Autodesk Inventor part; units mm, degrees
ref_plane "YZ Plane" through (0, 0, 0) normal (1, 0, 0) x (0, 1, 0)
ref_plane "XZ Plane" through (0, 0, 0) normal (0, 1, 0) x (-1, 0, 0)
ref_plane "XY Plane" through (0, 0, 0) normal (0, 0, 1) x (1, 0, 0)
sketch "Sketch1" plane through (0, 0, 0) normal (0, 0, 1) x (1, 0, 0)
  arc A0 (-3.1, 0) -> (3.1, 0) centre (0, 0) ccw
  arc A1 (-5.5, 0) -> (5.5, 0) centre (0, 0) ccw
  line L0 (-3.1, 0) -> (-5.5, 0)
  line L1 (-5.5, 0) -> (-5.5, 5.5)
  line L2 (-5.5, 5.5) -> (-3.1, 5.5)
  line L3 (-3.1, 5.5) -> (-3.1, 0)
  line L4 (3.1, 0) -> (5.5, 0)
  line L5 (5.5, 0) -> (5.5, 5.5)
  line L6 (5.5, 5.5) -> (3.1, 5.5)
  line L7 (3.1, 5.5) -> (3.1, 0)
  line L8 (-5.5, 0) -> (-5.5, 5.5)
  line L9 (-5.5, 5.5) -> (-17.5, 5.5)
  line L10 (-17.5, 5.5) -> (-17.5, 0)
  line L11 (-17.5, 0) -> (-5.5, 0)
  line L12 (5.5, 0) -> (5.5, 5.5)
  line L13 (5.5, 5.5) -> (17.5, 5.5)
  line L14 (17.5, 5.5) -> (17.5, 0)
  line L15 (17.5, 0) -> (5.5, 0)
  line L16 (17.5, 0) -> (17.5, -5.5)
  line L17 (17.5, -5.5) -> (-17.5, -5.5)
  line L18 (-17.5, -5.5) -> (-17.5, 0)
  dimension "d0" = 6.2
  dimension "d1" = 11
  dimension "d2" = 12
  dimension "d3" = 12
extrude "Extr-legs" add sketch "Sketch1" along normal blind 90 contours L11 L10 L9 L1 | L5 L13 L14 L15
extrude "Extr-base" add sketch "Sketch1" against normal blind 5 contours A0 L4 A1 L0 | L0 L1 L2 L3 | L7 L6 L5 L4 | L11 L10 L9 L1 | L5 L13 L14 L15
sketch "Sketch2" plane through (0, 0, 90) normal (0, 0, 1) x (1, 0, 0)
  circle A0 centre (0, 0) radius 2.2
  circle A1 centre (0, 0) radius 4.5
  line L0 (5.5, 0) -> (17.5, 0)
  line L1 (-17.5, 0) -> (-5.5, 0)
  line L2 (-17.5, 0) -> (-17.5, 5.5)
  line L3 (-17.5, 5.5) -> (17.5, 5.5)
  line L4 (17.5, 5.5) -> (17.5, 0)
  line L5 (17.5, 0) -> (2.2, 0)
  line L6 (-2.2, 0) -> (-17.5, 0)
  line L7 (-17.5, 0) -> (-17.5, -4.5048)
  line L8 (-17.5, -4.5048) -> (17.5, -4.5048)
  line L9 (17.5, -4.5048) -> (17.5, 0)
  line L10 (17.5, 0) -> (5.5, 0)
  line L11 (17.5, 0) -> (-1.5, 0)
  line L12 (-1.5, 0) -> (-1.5, -4.5048)
  line L13 (-1.5, -4.5048) -> (17.5, -4.5048)
  line L14 (17.5, -4.5048) -> (17.5, 0)
  line L15 (-17.5, 0) -> (-12.5, 0)
  line L16 (-12.5, 0) -> (-12.5, -4.5048)
  line L17 (-12.5, -4.5048) -> (-17.5, -4.5048)
  line L18 (-17.5, -4.5048) -> (-17.5, 0)
  dimension "d8" = 4.4
  dimension "d9" = 9
extrude "Extr-top" add sketch "Sketch2" along normal blind 5 contours L5 A1 L12 A0 | A0 L6 A1 L5 | A0 L12 A1 L6 | L5 L0 L9 L8 L12 A1 | A1 L6 L1 L2 L3 L4 L0 L5 | A1 L12 L8 L16 L1 L6 | L16 L8 L7 L1
extrude "Extrusion4" add sketch "Sketch1" against normal up to surface (5 mm away) contours A1 L17 L18 L11 | L15 L16 L17 A1
sketch "Sketch3" plane through (0, 0, 90) normal (0, 0, -1) x (-1, 0, 0)
  line L0 (-5.5, 0) -> (-17.5, 0)
  line L1 (-17.5, -4.5048) -> (-17.5, 0)
  line L2 (17.5, -4.5048) -> (-17.5, -4.5048)
  line L3 (17.5, 0) -> (17.5, -4.5048)
  line L4 (17.5, 0) -> (5.5, 0)
  line L5 (5.5, 0) -> (5.5, 5.5)
  line L6 (-5.5, 5.5) -> (5.5, 5.5)
  line L7 (-5.5, 5.5) -> (-5.5, 0)
  circle A0 centre (0, 0) radius 2.2
  line L8 (17.5, -4.5048) -> (-17.5, -4.5048)
  line L9 (-17.5, 0) -> (-5.5, 0)
  line L10 (-5.5, 0) -> (-5.5, -4.5048)
  line L11 (-5.5, -4.5048) -> (-17.5, -4.5048)
  line L12 (-17.5, -4.5048) -> (-17.5, 0)
  line L13 (17.5, 0) -> (5.5, 0)
  line L14 (5.5, 0) -> (17.5, 0)
  line L15 (17.5, 0) -> (17.5, -4.5048)
  line L16 (17.5, -4.5048) -> (5.5, -4.5048)
  line L17 (5.5, -4.5048) -> (5.5, 0)
extrude "Extrusion5" add sketch "Sketch3" along normal up to next contours L10 L2 L1 L0 | L17 L4 L3 L2
sketch "Sketch4" plane through (0, 0, 0) normal (0, 0, 1) x (1, 0, 0)
  line L0 (-17.5, -5.5) -> (17.5, -5.5)
  line L1 (-5.5, -4.5048) -> (-17.5, -4.5048)
  line L2 (-17.5, -5.5) -> (-5.5, -5.5)
  line L3 (-5.5, -5.5) -> (-5.5, -4.5048)
  line L4 (-5.5, -4.5048) -> (-17.5, -4.5048)
  line L5 (-17.5, -4.5048) -> (-17.5, -5.5)
  line L6 (17.5, -4.5048) -> (5.5, -4.5048)
  line L7 (-17.5, -5.5) -> (17.5, -5.5)
  line L8 (17.5, -4.5048) -> (5.5064, -4.5048)
  line L9 (5.5064, -4.5048) -> (5.5064, -5.5)
  line L10 (5.5064, -5.5) -> (17.5, -5.5)
  line L11 (17.5, -5.5) -> (17.5, -4.5048)
  point P0 (0, 0)
extrude "Extrusion6" add sketch "Sketch4" along normal up to surface (95 mm away)
sketch "Sketch5" plane through (0, 0, 95) normal (0, 0, 1) x (1, 0, 0)
  line L0 (-5.5, -4.5048) -> (5.5, -4.5048)
  line L1 (-17.5, -5.5) -> (17.5, -5.5)
  line L2 (-5.5, -4.5048) -> (5.516, -4.5048)
  line L3 (5.516, -4.5048) -> (5.516, -5.5)
  line L4 (5.516, -5.5) -> (-5.5, -5.5)
  line L5 (-5.5, -5.5) -> (-5.5, -4.5048)
  point P0 (0, 0)
extrude "Extrusion7" add sketch "Sketch5" against normal up to surface (5 mm away)
properties part number "cage2table-mount-M4(top)-M6(bottom)-H100mm"
Model file for the job. Use its own axes, mm. A direction names the side the tool comes from. Give positions to 0.01 mm unless a question says otherwise; leave off trailing zeros. Loops run counter-clockwise (first coordinate to the right, second up) from the corner with the lowest first, then second, coordinate; pieces in that order, holes last. Notation, with made-up numbers: M -21.5,55 L 30.5,55 A13 ccw 30.5,74 Z; hole C -5,20 d1. An arc over 180 degrees is marked long. Use one line per item in the form item = value.
Item 1: Drill centre lines: L1, parallel to Y at x = 0, z = 93; L2, parallel to X at y = -4, z = 89.5; L3, parallel to X at y = 0, z = 93.35. Where is each one in solid material? Low to high.
Filled in:
L1 = -5.5 to -2.2, 2.2 to 5.5
L2 = -17.5 to -5.5, 5.5 to 17.5
L3 = -17.5 to -2.2, 2.2 to 17.5
Item 2: Flat gauge pin, fed straight in: pin 1 Ø6 at (x, z) = (1.5, 72.5) entering from -Y. Where does the tip first touch, or does it go through?
Filled in:
pin_1 = through
Item 3: Slice it at C-C on x = 0. List the corners of the cut face in (y, z).
Filled in:
outline = M -5.5,-5 L -3.1,-5 L -3.1,0 L -5.5,0 Z; M -5.5,90 L -2.2,90 L -2.2,95 L -5.5,95 Z; M 2.2,90 L 5.5,90 L 5.5,95 L 2.2,95 Z
Item 4: Slice it at B-B on x = -4. List the corners of the cut face in (y, z), and give its area (3 significant figures).
Filled in:
outline = M -5.5,-5 L 5.5,-5 L 5.5,0 L -5.5,0 Z; M -5.5,90 L 5.5,90 L 5.5,95 L -5.5,95 Z
area = 110 mm^2
Item 5: Which spindle directions (+Z, -Z, +X, -X, +Y, -Y) get a long thin tool onto all of the face, cutting with end or side? Do faces 1 (the flat face through (3.1, 3, -2)), 2 (the flat face through (-5.5, 0, 44)), 3 (the flat face through (8, -5.5, 46)). Say none if no direction does.
Filled in:
face_1 = -Z, +Y
face_2 = +Y, -Y
face_3 = +Z, -Z, +X, -X, -Y
Item 6: Two-plate mould, pull along Z, no slides. Class faces 4 (the flat face through (-8, 5.5, 44)), 5 (the flat face through (0, 3, 95)), 6 (the flat face through (5.5, 0, 44)): released by +Z, released by -Z, zero draft, split by the parting line, or undercut.
Filled in:
face_4 = zero draft
face_5 = released by +Z
face_6 = undercut
